from build123d import *

# Parameters (mm, degrees)
PAD002_DEPTH    = 5.55
POCKET001_DEPTH = 0.5
POCKET002_DEPTH = 0.5
PAD003_DEPTH    = 2.5
PAD001_DEPTH    = 9
SKETCH_R        = 9
PAD_DEPTH       = 11.8
SKETCH001_R     = 11.05
POCKET_DEPTH    = 10
SKETCH010_R     = 1.6
POCKET003_DEPTH = 5
FILLET_R        = 1.8
SKETCH011_R     = 2.1
POCKET004_DEPTH = 5
POCKET005_DEPTH = 2
FILLET001_R     = 2


with BuildPart() as pad003:
    # Sketch004 → Pad002 (new body)
    with BuildSketch(Plane.XY.offset(2.225)):
        Polygon((-11.1717282118, -2.7499991288), (-7.9674332118, -8.3000008712), (-8.4004459137, -8.5500008712), (-11.6047409137, -2.9999991288), align=None)
    extrude(amount=PAD002_DEPTH)

    # Sketch006 → Pocket001 (cut)
    with BuildSketch(Plane(origin=(-9.5695807118, -5.525, 2.225), x_dir=(-0.5, 0.8660254038, 0), z_dir=(0.8660254038, 0.5, 0))):
        Polygon((-3.204295, 2.7750019602), (-1.6021491347, 5.55), (-3.204295, 5.55), align=None)
        Polygon((1.6021478772, 0), (3.204295, 0), (3.204295, 2.7750019602), align=None)
    extrude(amount=-POCKET001_DEPTH, mode=Mode.SUBTRACT)

    # Sketch008 → Pocket002 (cut)
    with BuildSketch(Plane(origin=(-9.5695807118, -5.525, 2.225), x_dir=(-0.5, 0.8660254038, 0), z_dir=(0.8660254038, 0.5, 0))):
        Polygon((1.6021478772, 5.5500030493), (3.204295, 5.5500030493), (3.204295, 2.7750019602), align=None)
        Polygon((-1.6021478772, 0), (-3.2042957545, 0), (-3.2042957545, 2.7750015246), align=None)
    extrude(amount=-POCKET002_DEPTH, mode=Mode.SUBTRACT)

    # Sketch009 → Pad003 (new body, symmetric)
    with BuildSketch(Plane(origin=(-9.5695807118, -5.525, 2.225), x_dir=(-0.5, 0.8660254038, 0), z_dir=(0.8660254038, 0.5, 0))):
        Polygon((1.6021491347, -7.4054e-06), (3.2042982695, 2.7749962973), (1.6021491347, 5.55), (-1.6021491347, 5.55), (-3.2042982695, 2.7749962973), (-1.6021491347, -7.4054e-06), align=None)
    extrude(amount=PAD003_DEPTH, both=True)


with BuildPart() as pad001:
    # Sketch003 → Pad001 (new body)
    with BuildSketch(Plane.XY):
        with BuildLine():
            ThreePointArc((-10.9554657182, -1.442314424), (-9.5695807118, -5.525), (-6.7268137905, -8.7665544102))
            Line((-9.4662402211, -12.3366444415), (-6.7268137905, -8.7665544102))
            ThreePointArc((-15.4169675944, -2.029682289), (-13.4666950288, -7.775), (-9.4662402211, -12.3366444415))
            Line((-10.9554657182, -1.442314424), (-15.4169675944, -2.029682289))
        make_face()
    extrude(amount=PAD001_DEPTH)


with BuildPart() as fillet001:
    # Sketch → Pad (new body)
    with BuildSketch(Plane.XY):
        with BuildLine():
            Line((-23, 11.5), (23, 11.5))
            Line((23, 11.5), (23, 7.5))
            Line((23, 7.5), (15, 7.5))
            ThreePointArc((15, 7.5), (13.217253485, 6.6833607789), (12.6713258975, 4.8))
            ThreePointArc((-12.6713258975, 4.8), (0, -13.55), (12.6713258975, 4.8))
            ThreePointArc((-12.6713258975, 4.8), (-13.217253485, 6.6833607789), (-15, 7.5))
            Line((-15, 7.5), (-23, 7.5))
            Line((-23, 7.5), (-23, 11.5))
        make_face()
        Circle(SKETCH_R, mode=Mode.SUBTRACT)
    extrude(amount=PAD_DEPTH)

    # Sketch001 → Pocket (cut)
    with BuildSketch(Plane.XY.offset(11.8)):
        Circle(SKETCH001_R)
    extrude(amount=-POCKET_DEPTH, mode=Mode.SUBTRACT)

    # Fusion: union Pad001
    add(pad001.part)

    # Cut: cut Pad003
    add(pad003.part, mode=Mode.SUBTRACT)

    # Sketch010 → Pocket003 (cut)
    with BuildSketch(Plane(origin=(-11.7346442213, -6.775, 0), x_dir=(-0.5, 0.8660254038, 0), z_dir=(0.8660254038, 0.5, 0))):
        with Locations((0, 4.9999962973)):
            Circle(SKETCH010_R)
    extrude(amount=-POCKET003_DEPTH, mode=Mode.SUBTRACT)

    # Fillet
    fillet_edges = [fillet001.edges().sort_by_distance(p)[0] for p in [
        (-15.416968, -2.029682, 4.5),
        (-9.46624, -12.336644, 4.5),
    ]]
    fillet(fillet_edges, radius=FILLET_R)

    # Sketch011 → Pocket004 (cut)
    with BuildSketch(Plane.XZ.offset(-7.5)):
        with Locations((-18.5, 5.9)):
            Circle(SKETCH011_R)
        with Locations((18.5, 5.9)):
            Circle(SKETCH011_R)
    extrude(amount=-POCKET004_DEPTH, mode=Mode.SUBTRACT)

    # Sketch012 → Pocket005 (cut, symmetric)
    with BuildSketch(Plane.XZ.offset(-7.5)):
        Polygon((-20.5351596989, 2.375), (-16.4648403011, 2.375), (-14.4296806022, 5.9), (-16.4648403011, 9.425), (-20.5351596989, 9.425), (-22.5703193978, 5.9), align=None)
        Polygon((16.4648403011, 2.375), (20.5351596989, 2.375), (22.5703193978, 5.9), (20.5351596989, 9.425), (16.4648403011, 9.425), (14.4296806022, 5.9), align=None)
    extrude(amount=POCKET005_DEPTH, both=True, mode=Mode.SUBTRACT)

    # Fillet001
    fillet001_edges = [fillet001.edges().sort_by_distance(p)[0] for p in [
        (-23, 9.5, 0),
        (-23, 9.5, 11.8),
        (23, 9.5, 0),
        (23, 9.5, 11.8),
    ]]
    fillet(fillet001_edges, radius=FILLET001_R)


solid = fillet001.part
The model under review builds one solid part; all positions refer to its coordinate system, in mm. A direction names the side the tool comes from. Give positions to 0.01 mm unless a question says otherwise; leave off trailing zeros. Order: outer loops, then holes, each group sorted by start corner. A loop starts at its lowest first (then second) coordinate and runs counter-clockwise, first axis right, second up. Notation, with made-up numbers: M 62.25,59 L 120.25,59 A30 cw 120.25,83 Z; hole C 35.5,-5.5 d3. An arc over 180 degrees is marked long. One line per question, with ' | ' between items. Start each with the question number.
1) Consider section B-B, the plane x = 0. Give the boundary of the cut face in (y, z), then the cut area to 3 significant figures.
2) Wall thickness on L1, parallel to Y at x = 0.5, z = 7.25; L2, parallel to X at y = 0, z = 0.65; L3, parallel to X at y = 2.5, z = 10.25: over which ranges is each line inside the solid? List them lowest first. Write a range as from..to.
3) Consider section A-A, the plane y = 0. Give the boundary of the cut face in (x, z).
4) Mouldability with a two-part tool opening along Y and no side actions: class faces 4 (the face through (22, 7.5, 3)), 5 (the face through (-11.95, -8.37, 4.03)), 6 (the face through (-9.22, -8.11, 3.63)), 7 (the face through (-19, 9, 2.375)) as pulls with the +Y half, pulls with the -Y half, needs draft (parallel to the pull), parting line crosses it, or undercut.
5) For faces 1 (the face through (-15.433, 8.479, 7.638)), 2 (the face through (-12, -7, 9)), 3 (the face through (21.538, 8.486, 4.113)), list the 3-axis set-ups (+Z, -Z, +X, -X, +Y, -Y) from which the entire face can be reached by the end or side of a thin tool; tool diameter is ignored.
6) Clearance check with flat-ended pins moving along their axes: P1, Ø4, axis at y = -7.5, z = 2, coming from the -X side; P2, Ø6.5, axis at x = 18, z = 3.5, coming from the -Y side; P3, Ø6, axis at y = -9, z = 5, coming from the -X side. State where each tip first meets the part, or that it passes through.
Found:
1) outline: M -13.55,0 L -9,0 L -9,1.8 L -11.05,1.8 L -11.05,11.8 L -13.55,11.8 Z; M 9,0 L 11.5,0 L 11.5,11.8 L 11.05,11.8 L 11.05,1.8 L 9,1.8 Z | area: 42.2 mm²
2) L1: y = -13.54..-11.04, 11.04..11.5 | L2: x = -13.55..-9, 9..13.55 | L3: x = -13.32..-10.76, 10.76..13.32
3) outline: M -13.55,0 L -9,0 L -9,1.8 L -11.05,1.8 L -11.05,11.8 L -13.55,11.8 Z; M 9,0 L 13.55,0 L 13.55,11.8 L 11.05,11.8 L 11.05,1.8 L 9,1.8 Z
4) face 4: pulls with the -Y half | face 5: undercut | face 6: undercut | face 7: needs draft
5) face 1: none | face 2: +Z, -X, -Y | face 3: -Y
6) P1: stops at x = -14.54 | P2: stops at y = 7.49 | P3: stops at x = -14.35
